```python
from build123d import *

# Parameters (mm, degrees)
SKETCH_1_W          = 40
SKETCH_1_H          = 43
SKETCH_1_R          = 1.8
EXTRUDE_1_DEPTH     = 3
SKETCH_2_W          = 40
SKETCH_2_H          = 3
EXTRUDE_2_DEPTH     = 44
SKETCH_3_R          = 1.6
CUT_EXTRUDE_1_DEPTH = 44
FILLET_1_R          = 20
FILLET_2_R          = 3
FILLET_3_R          = 3
FILLET_4_R          = 3


with BuildPart() as part:
    # 草图1 → 凸台-拉伸1 (new body)
    with BuildSketch(Plane(origin=(0, 0, 0), x_dir=(1, 0, 0), z_dir=(0, 1, 0))):
        Rectangle(SKETCH_1_W, SKETCH_1_H)
        with Locations(Location((-15, 13.5, 0), (0, 0, 270))):
            Circle(SKETCH_1_R, mode=Mode.SUBTRACT)
        with Locations(Location((15, 13.5, 0), (0, 0, 270))):
            Circle(SKETCH_1_R, mode=Mode.SUBTRACT)
        with Locations(Location((15, -10.5, 0), (0, 0, 270))):
            Circle(SKETCH_1_R, mode=Mode.SUBTRACT)
        with Locations(Location((-15, -10.5, 0), (0, 0, 270))):
            Circle(SKETCH_1_R, mode=Mode.SUBTRACT)
    extrude(amount=EXTRUDE_1_DEPTH)

    # 草图2 → 凸台-拉伸2 (add)
    with BuildSketch(Plane(origin=(0, 3, 0), x_dir=(1, 0, 0), z_dir=(0, 1, 0))):
        with Locations((0, -20)):
            Rectangle(SKETCH_2_W, SKETCH_2_H)
    extrude(amount=EXTRUDE_2_DEPTH)

    # 草图3 → 切除-拉伸1 (cut)
    with BuildSketch(Plane(origin=(0, 0, 18.5), x_dir=(-1, 0, 0), z_dir=(0, 0, -1))):
        with Locations((15.5, 25.5)):
            Circle(SKETCH_3_R)
        with Locations((-15.5, 25.5)):
            Circle(SKETCH_3_R)
        with Locations((-7.75, 38.923393759)):
            Circle(SKETCH_3_R)
        with Locations((-7.75, 12.076606241)):
            Circle(SKETCH_3_R)
        with Locations((7.75, 12.076606241)):
            Circle(SKETCH_3_R)
        with Locations((7.75, 38.923393759)):
            Circle(SKETCH_3_R)
        with BuildLine():
            Line((6.5, 32.5), (6.5, 18.5))
            ThreePointArc((6.5, 18.5), (0, 12), (-6.5, 18.5))
            Line((-6.5, 18.5), (-6.5, 32.5))
            ThreePointArc((-6.5, 32.5), (0, 39), (6.5, 32.5))
        make_face()
    extrude(amount=-CUT_EXTRUDE_1_DEPTH, mode=Mode.SUBTRACT)

    # 圆角1
    fillet_1_edges = [part.edges().sort_by_distance(p)[0] for p in [
        (-20, 47, 20),
        (20, 47, 20),
    ]]
    fillet(fillet_1_edges, radius=FILLET_1_R - 0.0001)  # a hair under: the kernel refuses the full size

    # 圆角2
    fillet_2_edges = [part.edges().sort_by_distance(p)[0] for p in [
        (20, 1.5, -21.5),
    ]]
    fillet(fillet_2_edges, radius=FILLET_2_R)

    # 圆角3
    fillet_3_edges = [part.edges().sort_by_distance(p)[0] for p in [
        (-20, 1.5, -21.5),
    ]]
    fillet(fillet_3_edges, radius=FILLET_3_R)

    # 圆角4
    fillet_4_edges = [part.edges().sort_by_distance(p)[0] for p in [
        (0, 0, 21.5),
    ]]
    fillet(fillet_4_edges, radius=FILLET_4_R)


solid = part.part
```
Check sheet for the modelled part. Datum: model origin and axes. Units: mm. A direction names the side the tool comes from. Coordinates: 2 decimals unless noted, no trailing zeros. Loops run counter-clockwise (first coordinate to the right, second up) from the corner with the lowest first, then second, coordinate; pieces in that order, holes last. Notation, with made-up numbers: M -31.75,-20.75 L 9.25,-20.75 A17 ccw 9.25,10.25 Z; hole C 0,-32 d8. An arc over 180 degrees is marked long. Answer as a JSON object with one key per item and string values.
1. Release check for a two-part mould opening along X. For faces 3 (the flat face through (9, 25, 18.5)), 4 (the cylindrical face through (13.986, 41.297, 19.979)), 5 (the flat face through (-6.5, 26, 20)) record: pulls with the +X half, pulls with the -X half, needs draft (parallel to the pull), parting line crosses it, or undercut.
Outcome:
{"face 3": "needs draft", "face 4": "pulls with the +X half", "face 5": "undercut"}
2. Sectioned sample at A-A on y = 25.5. Record the cut outline in (x, z).
Outcome:
{"outline": "M -20,18.5 L -17.1,18.5 L -17.1,21.5 L -20,21.5 Z; M -13.9,18.5 L -6.5,18.5 L -6.5,21.5 L -13.9,21.5 Z; M 6.5,18.5 L 13.9,18.5 L 13.9,21.5 L 6.5,21.5 Z; M 17.1,18.5 L 20,18.5 L 20,21.5 L 17.1,21.5 Z"}
3. Depth check by flat-ended pin: P1, Ø3, axis at x = 15, z = 10.5, coming from the +Y side; P2, Ø5, axis at x = -7, z = -1, coming from the +Y side; P3, Ø4, axis at x = -7.75, y = 12.08, coming from the -Z side. Enter the tip coordinate at first touch or a pass-through.
Outcome:
{"P1": "through", "P2": "y = 3", "P3": "z = 18.5"}
4. Scan lines: L1, parallel to X at y = 2.4, z = -13.5; L2, parallel to Y at x = -7.75, z = 20.1; L3, parallel to Y at x = -7.75, z = 20.7. Record each from-to range of solid material in increasing order. Write a range as from..to.
Outcome:
{"L1": "-20..-16.8, -13.2..13.2, 16.8..20", "L2": "0.46..10.48, 13.68..37.32, 40.52..45.44", "L3": "0.96..10.48, 13.68..37.32, 40.52..45.44"}
5. Sectioned sample at D-D on y = 33.5. Record the cut outline in (x, z), and give its area (4 significant figures).
Outcome:
{"outline": "M -18.91,18.5 L -6.42,18.5 L -6.42,21.5 L -18.91,21.5 Z; M 6.42,18.5 L 18.91,18.5 L 18.91,21.5 L 6.42,21.5 Z", "area": "74.95 mm²"}
6. Access from +Z, -Z, +X, -X, +Y, -Y to the whole of each face (thin tool, end or side, straight path). Record for faces 1 (the flat face through (6.5, 25, 20)), 2 (the flat face through (-20, 2, 9)).
Outcome:
{"face 1": "+Z, -Z", "face 2": "+Z, -Z, -X, +Y, -Y"}
7. Sectioned sample at C-C on z = 11. Record the cut outline in (x, y), and give its area (4 significant figures).
Outcome:
{"outline": "M -20,0 L -16.73,0 L -16.73,3 L -20,3 Z; M -13.27,0 L 13.27,0 L 13.27,3 L -13.27,3 Z; M 16.73,0 L 20,0 L 20,3 L 16.73,3 Z", "area": "99.25 mm²"}
8. Sectioned sample at B-B on x = 1. Record the cut outline in (y, z).
Outcome:
{"outline": "M 0,-21.5 L 3,-21.5 L 3,18.5 L 12.08,18.5 L 12.08,21.5 L 3,21.5 A3 ccw 0,18.5 Z; M 38.92,18.5 L 46.97,18.5 L 46.97,21.5 L 38.92,21.5 Z"}
